```python
from build123d import *

# Parameters (mm, degrees)
F0_W     = 2000
F0_H     = 1600
F1_DEPTH = 500
F2_W     = 400
F2_H     = 175
F3_DEPTH = 20
F4_W     = 545
F4_H     = 1500
F5_DEPTH = 15


with BuildPart() as f1:
    # F0 (on Front) → F1 (new body)
    with BuildSketch(Plane.XZ):
        with Locations((1000, 800)):
            Rectangle(F0_W, F0_H)
    extrude(amount=F1_DEPTH)

    # F2 (on face) → F3 (cut)
    with BuildSketch(Plane.XZ.offset(500)):
        with Locations((1600, 1182.5)):
            Rectangle(F2_W, F2_H)
    extrude(amount=-F3_DEPTH, mode=Mode.SUBTRACT)

    # F4 (on face) → F5 (cut)
    with BuildSketch(Plane.XZ.offset(500)):
        with Locations((347.5, 795)):
            Rectangle(F4_W, F4_H)
        with Locations((967.5, 795)):
            Rectangle(F4_W, F4_H)
    extrude(amount=-F5_DEPTH, mode=Mode.SUBTRACT)


solid = f1.part
```
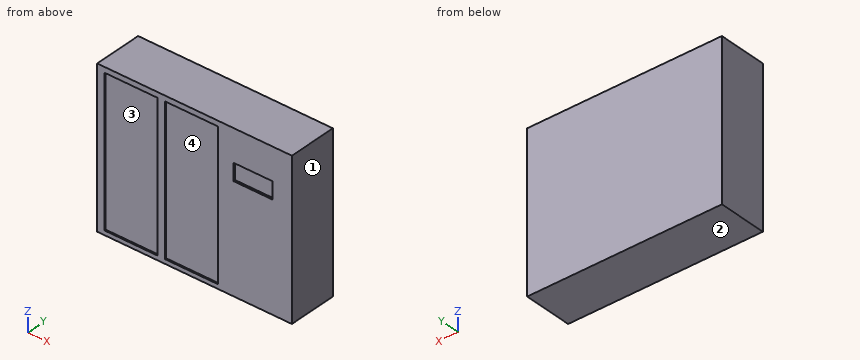
Work out the finished part from the listing and answer in its coordinate system (mm). Face numbers are marked on the shaded views. Give positions to 0.01 mm unless a question says otherwise; leave off trailing zeros. Loops run counter-clockwise (first coordinate to the right, second up) from the corner with the lowest first, then second, coordinate; pieces in that order, holes last. Notation, with made-up numbers: (67, 78) - (126, 78) arc R4 cw to (126, 82) - close; hole circle Ø11 at (56.5, -17). An arc over 180 degrees is marked (long way). One line per question, with ' | ' between items.
(1) A straight line is drawn through the part: probe 1 along Y at (x, z) = (1130, 1387). Find the intervals that lie inside material, in ascending order.
Recorded:
probe 1: y = -485 to 0
(2) The part is cut by section A-A (z = 159). Write down the section's boundary in (x, y).
Recorded:
outline: (0, -500) - (75, -500) - (75, -485) - (620, -485) - (620, -500) - (695, -500) - (695, -485) - (1240, -485) - (1240, -500) - (2000, -500) - (2000, 0) - (0, 0) - close
(3) The mould has two halves that part along Z. Classify the marked faces 1, 2, 3 and 4: +Z half, -Z half, draft (parallel to the pull), parting line (faces both ways), or undercut.
Recorded:
face 1: draft | face 2: -Z half | face 3: undercut | face 4: undercut
(4) The part is cut by section B-B (x = 162.5). Write down the section's boundary in (y, z), then the cut area to 4 significant figures.
Recorded:
outline: (-500, 0) - (0, 0) - (0, 1600) - (-500, 1600) - (-500, 1545) - (-485, 1545) - (-485, 45) - (-500, 45) - close | area: 777,500 mm²
(5) This flat-tipped pin is pushed along its axis until it touches: pin 1 Ø6 at (x, z) = (1070.5, 305) entering from -Y. Where does it stop, or does it pass through?
Recorded:
pin 1: stops at y = -485
